```python
from build123d import *

# Parameters (mm, degrees)
SKETCH1_R           = 1.5
SKETCH1_W           = 48.470262398
SKETCH1_H           = 3.779033876
BOSS_EXTRUDE1_DEPTH = 1.5


with BuildPart() as part:
    # Sketch1 → Boss-Extrude1 (new body)
    with BuildSketch(Plane(origin=(0, 0, 0), x_dir=(1, 0, 0), z_dir=(0, 1, 0))):
        with BuildLine():
            Line((29.5, -15), (-29.5, -15))
            ThreePointArc((-29.5, -15), (-31.621320344, -14.121320344), (-32.5, -12))
            Line((-32.5, -12), (-32.5, 12))
            ThreePointArc((-32.5, 12), (-31.621320344, 14.121320344), (-29.5, 15))
            Line((-29.5, 15), (29.5, 15))
            ThreePointArc((29.5, 15), (31.621320344, 14.121320344), (32.5, 12))
            Line((32.5, 12), (32.5, -12))
            ThreePointArc((32.5, -12), (31.621320344, -14.121320344), (29.5, -15))
        make_face()
        with Locations(Location((-29, 11.5, 0), (0, 0, 270))):
            Circle(SKETCH1_R, mode=Mode.SUBTRACT)
        with Locations(Location((29, 11.5, 0), (0, 0, 270))):
            Circle(SKETCH1_R, mode=Mode.SUBTRACT)
        with Locations(Location((29, -11.5, 0), (0, 0, 270))):
            Circle(SKETCH1_R, mode=Mode.SUBTRACT)
        with Locations(Location((-29, -11.5, 0), (0, 0, 270))):
            Circle(SKETCH1_R, mode=Mode.SUBTRACT)
        with Locations((0, 11.5)):
            Rectangle(SKETCH1_W, SKETCH1_H, mode=Mode.SUBTRACT)
    extrude(amount=BOSS_EXTRUDE1_DEPTH)


solid = part.part
```
Can you work these out from the model? Positions are in its coordinate system, mm. A direction names the side the tool comes from. Coordinates: 2 decimals unless noted, no trailing zeros. Loops run counter-clockwise (first coordinate to the right, second up) from the corner with the lowest first, then second, coordinate; pieces in that order, holes last. Notation, with made-up numbers: (79.25, 21) - (109.25, 21) arc R16 ccw to (109.25, 31) - close; hole circle Ø2 at (-6, 56.5). An arc over 180 degrees is marked (long way). Use a Markdown table: item, result.
Item 1: We'd pull the mould along Z, two halves only. Please class faces 3 (the face through (31.6, 0.74, -14.14)), 4 (the face through (-24.235, 1, -11)), 5 (the face through (32.5, 1, 0)): released by +Z, released by -Z, zero draft, split by the parting line, or undercut.
Numbers:
| item | result |
|---|---|
| face 3 | released by -Z |
| face 4 | undercut |
| face 5 | zero draft |
Item 2: I want a section at B-B on x = -10. Please give me the cut outline in (y, z).
Numbers:
| item | result |
|---|---|
| outline | (0, -15) - (1.5, -15) - (1.5, -13.39) - (0, -13.39) - close; (0, -9.61) - (1.5, -9.61) - (1.5, 15) - (0, 15) - close |
Item 3: If I drill on probe 1 along X at (y, z) = (0.85, -11.5); probe 2 along X at (y, z) = (1.15, 11.5); probe 3 along Z at (x, y) = (9, 1.4), over which ranges is the centre line in solid material (lowest first)? Write a range as from..to.
Numbers:
| item | result |
|---|---|
| probe 1 | x = -32.5..-30.5, -27.5..-24.24, 24.24..27.5, 30.5..32.5 |
| probe 2 | x = -32.5..-30.5, -27.5..27.5, 30.5..32.5 |
| probe 3 | z = -15..-13.39, -9.61..15 |
Item 4: For faces 1 (the face through (31.64, 0.74, 14.1)), 2 (the face through (0, 1, -13.39)), which set-ups out of +Z, -Z, +X, -X, +Y, -Y let a thin tool reach every point of the face, with its end or its side?
Numbers:
| item | result |
|---|---|
| face 1 | +Z, +X, +Y, -Y |
| face 2 | +Y, -Y |
Item 5: I want a section at A-A on y = 1.25. Please give me the cut outline in (x, z).
Numbers:
| item | result |
|---|---|
| outline | (-32.5, -12) arc R3 ccw to (-29.5, -15) - (29.5, -15) arc R3 ccw to (32.5, -12) - (32.5, 12) arc R3 ccw to (29.5, 15) - (-29.5, 15) arc R3 ccw to (-32.5, 12) - close; hole circle Ø3 at (-29, -11.5); hole circle Ø3 at (-29, 11.5); hole (-24.24, -13.39) - (24.24, -13.39) - (24.24, -9.61) - (-24.24, -9.61) - close; hole circle Ø3 at (29, -11.5); hole circle Ø3 at (29, 11.5) |
